Autodesk Fusion 360 part; units mm, degrees
sketch "podklad" plane through (0, 0, 0) normal (0, 1, 0) x (1, 0, 0)
  line L0 (45, -67.4927) -> (75, -67.4927) construction
  line L1 (-75.0372, -23.4927) -> (-85, -23.4927)
  arc A0 (96.7123, 33.4364) -> (98.5902, 36.1245) centre (96.7123, 35.4364) ccw
  line L2 (45, -38.4927) -> (45, -67.4927) construction
  line L3 (85, -33.4277) -> (85, -23.4927)
  line L4 (-75.0372, -23.4927) -> (-75.0372, 23.5073)
  line L5 (74.9628, -23.4927) -> (74.9628, 23.5073)
  line L6 (0, 105) -> (0, -105) construction
  line L7 (-85, 23.5073) -> (-75.0372, 23.5073)
  arc A1 (-98.5902, 36.1245) -> (-96.7123, 33.4364) centre (-96.7123, 35.4364) ccw
  arc A2 (-96.7154, -33.4277) -> (-98.5934, -36.1156) centre (-96.7154, -35.4277) ccw
  line L8 (74.9628, -23.4927) -> (85, -23.4927)
  line L9 (85, 23.5073) -> (74.9628, 23.5073)
  line L10 (-85, 33.4364) -> (-85, 23.5073)
  arc A3 (-98.5934, -36.1156) -> (98.5934, -36.1156) centre (0, 0) ccw
  line L11 (85, 33.4364) -> (85, 23.5073)
  line L12 (96.7123, 33.4364) -> (85, 33.4364)
  line L13 (-96.7154, -33.4277) -> (-85, -33.4277)
  arc A4 (98.5934, -36.1156) -> (96.7154, -33.4277) centre (96.7154, -35.4277) ccw
  line L14 (75, -67.4927) -> (75, -38.4927) construction
  arc A5 (98.5902, 36.1245) -> (15, 103.923) centre (0, 0) ccw
  arc A6 (15, 103.923) -> (-15, 103.923) centre (0, 0) ccw
  arc A7 (-15, 103.923) -> (-98.5902, 36.1245) centre (0, 0) ccw
  circle A8 centre (75, -38.4927) radius 1.1
  line L15 (75, -38.4927) -> (45, -38.4927) construction
  line L16 (-96.7123, 33.4364) -> (-85, 33.4364)
  circle A9 centre (75, -67.4927) radius 1.1
  circle A10 centre (45, -38.4927) radius 1.1
  line L17 (96.7154, -33.4277) -> (85, -33.4277)
  line L18 (-85, -33.4277) -> (-85, -23.4927)
  circle A11 centre (45, -67.4927) radius 1.1
  line L19 (51, -45) -> (69, -45)
  line L20 (70, -46) -> (70, -62)
  line L21 (69, -63) -> (51, -63)
  line L22 (50, -62) -> (50, -46)
  circle A12 centre (-30, -94.9953) radius 1.85
  circle A13 centre (30, -94.9953) radius 1.85
  circle A14 centre (-29.9934, 95.0047) radius 1.85
  circle A15 centre (29.9934, 95.0047) radius 1.85
  circle A16 centre (0, 0) radius 10
  circle A17 centre (-20, 0.003) radius 1.85
  circle A18 centre (-30, 0.0036) radius 1.85
  circle A19 centre (-40, 0.0023) radius 1.85
  circle A20 centre (-50, 0.0036) radius 1.85
  circle A21 centre (50, 0.0036) radius 1.85
  circle A22 centre (40, 0.0023) radius 1.85
  circle A23 centre (30, 0.0036) radius 1.85
  circle A24 centre (20, 0.003) radius 1.85
  arc A25 (51, -45) -> (50, -46) centre (51, -46) ccw
  arc A26 (70, -46) -> (69, -45) centre (69, -46) ccw
  arc A27 (69, -63) -> (70, -62) centre (69, -62) ccw
  arc A28 (50, -62) -> (51, -63) centre (51, -62) ccw
  line L23 (2.5, 0) -> (20, 0)
  line L24 (6, 15) -> (29, 15)
  line L25 (30, 16) -> (30, 74)
  line L26 (29, 75) -> (6, 75)
  line L27 (5, 74) -> (5, 16)
  arc A29 (6, 75) -> (5, 74) centre (6, 74) ccw
  arc A30 (30, 74) -> (29, 75) centre (29, 74) ccw
  arc A31 (29, 15) -> (30, 16) centre (29, 16) ccw
  arc A32 (5, 16) -> (6, 15) centre (6, 16) ccw
  line L28 (-56.6497, 57.6211) -> (-52.6497, 57.6211)
  line L29 (-52.6497, 33.6211) -> (-56.6497, 33.6211)
  line L30 (-56.6497, 33.6211) -> (-56.6497, 35.202)
  line L31 (-56.6497, 54.798) -> (-56.6497, 57.6211)
  line L32 (-52.6497, 57.6211) -> (-52.6497, 54.798)
  line L33 (-52.6497, 35.202) -> (-52.6497, 33.6211)
  arc A33 (-56.6497, 54.798) -> (-56.6497, 35.202) centre (-54.6497, 45) ccw
  arc A34 (-52.6497, 35.202) -> (-52.6497, 54.798) centre (-54.6497, 45) ccw
  point P0 (-7.5, -102.9967)
  point P1 (-82.0372, 22.8073)
  point P2 (-17.0372, -22.7927)
  point P3 (81.9628, 22.8073)
  point P4 (-0.0372, 0.0073)
  point P5 (-82.0372, -22.7927)
  point P6 (16.9628, 27.0073)
  point P7 (16.9628, 22.8073)
  point P8 (-17.0372, 27.0073)
  point P9 (16.9628, -22.7927)
  point P10 (81.9628, -22.7927)
  point P11 (16.9628, -26.9927)
  dimension "d1" = 210
  dimension "d2" = 2
  dimension "d3" = 2
  dimension "d4" = 2
  dimension "d5" = 2
  dimension "d26" = 30
  dimension "d27" = 29
  dimension "d28" = 2.2
  dimension "d29" = 2.2
  dimension "d30" = 2.2
  dimension "d31" = 2.2
  dimension "d32" = 45
  dimension "d33" = 15
  dimension "d39" = 3.7
  dimension "d40" = 20
  dimension "d41" = 3.7
  dimension "d42" = 3.7
  dimension "d43" = 3.7
  dimension "d44" = 20
  dimension "d45" = 30
  dimension "d46" = 40
  dimension "d47" = 3.7
  dimension "d48" = 50
  dimension "d49" = 1
  dimension "d50" = 1
  dimension "d51" = 1
  dimension "d52" = 1
  dimension "d74" = 1
  dimension "d75" = 20
  dimension "d76" = 4
  dimension "d77" = 24
  dimension "d78" = 2
extrude "Extrude1" add sketch "podklad" along normal blind 5
sketch "diry_hlavy_sroubu" plane through (0, 5, 0) normal (0, 1, 0) x (-1, 0, 0)
  circle A0 centre (29.9934, -95.0047) radius 1.85
  circle A1 centre (-29.9934, -95.0047) radius 1.85
  circle A2 centre (0, 0) radius 10
  circle A3 centre (40, -0.0023) radius 1.85
  circle A4 centre (-30, -0.0036) radius 1.85
  circle A5 centre (30, -0.0036) radius 1.85
  arc A6 (-51, 45) -> (-50, 46) centre (-51, 46) ccw
  line L0 (-51, 45) -> (-69, 45)
  arc A7 (-70, 46) -> (-69, 45) centre (-69, 46) ccw
  line L1 (-70, 46) -> (-70, 62)
  arc A8 (-69, 63) -> (-70, 62) centre (-69, 62) ccw
  line L2 (-69, 63) -> (-51, 63)
  arc A9 (-50, 62) -> (-51, 63) centre (-51, 62) ccw
  line L3 (-50, 62) -> (-50, 46)
  circle A10 centre (-45, 67.4927) radius 1.1
  circle A11 centre (-30, 94.9953) radius 1.85
  circle A12 centre (-50, -0.0036) radius 1.85
  circle A13 centre (-45, 38.4927) radius 1.1
  circle A14 centre (-75, 67.4927) radius 1.1
  circle A15 centre (50, -0.0036) radius 1.85
  circle A16 centre (30, 94.9953) radius 1.85
  circle A17 centre (-40, -0.0023) radius 1.85
  circle A18 centre (-20, -0.003) radius 1.85
  circle A19 centre (20, -0.003) radius 1.85
  circle A20 centre (-75, 38.4927) radius 1.1
  arc A21 (96.7154, 33.4277) -> (98.5934, 36.1156) centre (96.7154, 35.4277) ccw
  arc A22 (98.5934, 36.1156) -> (-98.5934, 36.1156) centre (0, 0) ccw
  arc A23 (-98.5934, 36.1156) -> (-96.7154, 33.4277) centre (-96.7154, 35.4277) ccw
  line L4 (-96.7154, 33.4277) -> (-85, 33.4277)
  line L5 (-85, 33.4277) -> (-85, 23.4927)
  line L6 (-85, 23.4927) -> (-74.9628, 23.4927)
  line L7 (-74.9628, 23.4927) -> (-74.9628, -23.5073)
  line L8 (-74.9628, -23.5073) -> (-85, -23.5073)
  line L9 (-85, -23.5073) -> (-85, -33.4364)
  line L10 (-85, -33.4364) -> (-96.7123, -33.4364)
  arc A24 (-96.7123, -33.4364) -> (-98.5902, -36.1245) centre (-96.7123, -35.4364) ccw
  arc A25 (-98.5902, -36.1245) -> (98.5902, -36.1245) centre (0, 0) ccw
  arc A26 (98.5902, -36.1245) -> (96.7123, -33.4364) centre (96.7123, -35.4364) ccw
  line L11 (96.7123, -33.4364) -> (85, -33.4364)
  line L12 (85, -33.4364) -> (85, -23.5073)
  line L13 (85, -23.5073) -> (75.0372, -23.5073)
  line L14 (75.0372, -23.5073) -> (75.0372, 23.4927)
  line L15 (75.0372, 23.4927) -> (85, 23.4927)
  line L16 (85, 23.4927) -> (85, 33.4277)
  line L17 (85, 33.4277) -> (96.7154, 33.4277)
  circle A27 centre (29.9934, -95.0047) radius 3.5
  circle A28 centre (-29.9934, -95.0047) radius 3.5
  circle A29 centre (30, 94.9953) radius 3.5
  circle A30 centre (-30, 94.9953) radius 3.5
  line L18 (-5, -16) -> (-5, -74)
  line L19 (-6, -75) -> (-29, -75)
  line L20 (-30, -74) -> (-30, -16)
  line L21 (-29, -15) -> (-6, -15)
  arc A31 (-5, -16) -> (-6, -15) centre (-6, -16) ccw
  arc A32 (-6, -75) -> (-5, -74) centre (-6, -74) ccw
  arc A33 (-30, -74) -> (-29, -75) centre (-29, -74) ccw
  arc A34 (-29, -15) -> (-30, -16) centre (-29, -16) ccw
  line L22 (52.6497, -35.202) -> (52.6497, -33.6211)
  line L23 (52.6497, -33.6211) -> (56.6497, -33.6211)
  line L24 (56.6497, -33.6211) -> (56.6497, -35.202)
  arc A35 (56.6497, -54.798) -> (56.6497, -35.202) centre (54.6497, -45) ccw
  line L25 (56.6497, -54.798) -> (56.6497, -57.6211)
  line L26 (56.6497, -57.6211) -> (52.6497, -57.6211)
  line L27 (52.6497, -57.6211) -> (52.6497, -54.798)
  arc A36 (52.6497, -35.202) -> (52.6497, -54.798) centre (54.6497, -45) ccw
  dimension "d55" = 7
  dimension "d56" = 7
  dimension "d57" = 7
  dimension "d58" = 7
extrude "Extrude3" cut sketch "diry_hlavy_sroubu" against normal blind 3 contours A27 | A28 | A29 | A30
sketch "sloupky_displej" plane through (0, 5, 0) normal (0, 1, 0) x (-1, 0, 0)
  circle A0 centre (-45, 38.4927) radius 4
  circle A1 centre (-75, 38.4927) radius 4
  circle A2 centre (-45, 67.4927) radius 4
  circle A3 centre (-75, 67.4927) radius 4
  circle A4 centre (-45, 67.4927) radius 1.1
  circle A5 centre (-75, 67.4927) radius 1.1
  circle A6 centre (-75, 38.4927) radius 1.1
  circle A7 centre (-45, 38.4927) radius 1.1
  point P0 (-45, 38.4927)
  point P1 (-75, 38.4927)
  point P2 (-45, 67.4927)
  point P3 (-75, 67.4927)
  point P4 (-43.9, 67.4927)
  point P5 (-73.9, 67.4927)
  point P6 (-73.9, 38.4927)
  point P7 (-43.9, 38.4927)
  dimension "d63" = 8
  dimension "d64" = 8
  dimension "d65" = 8
  dimension "d66" = 8
extrude "Extrude4" add sketch "sloupky_displej" along normal blind 5
Input: part model. Units: mm. Frame: model coordinates. A direction names the side the tool comes from. Give positions to 0.01 mm unless a question says otherwise; leave off trailing zeros. Write each loop counter-clockwise with the first axis right and the second up, starting at its lowest first coordinate (ties: lowest second). Pieces come first, ordered by that corner, then holes.
Q1. Pull-direction query (X, two-part tool) for faces 4 (the face through (91, 2, -33.436)), 5 (the face through (50, 2, 54)), 6 (the face through (85, 2, -29)); classes: pulls with the +X half, pulls with the -X half, needs draft (parallel to the pull), parting line crosses it, or undercut.
Q2. Section C-C, the plane y = 3.5. State how many separate pieces and enclosed holes the cut face has, plus the area to 3 significant figures.
Q3. Section A-A, the plane x = 0. Output: boundary loops of the cut face in (y, z), plus the area to 3 significant figures.
Q4. Material intervals for probe 1 along Z at (x, y) = (-30, 3.6); probe 2 along Z at (x, y) = (20.5, 1.75); probe 3 along X at (y, z) = (2.75, 68), sorted ascending.
Q5. First-contact query: P1, Ø2, axis at y = 1, z = -33.5, coming from the +X side; P2, Ø5, axis at y = 2, z = 75, coming from the +X side; P3, Ø4, axis at x = -81, y = 1.5, coming from the -Z side. Flat tips, straight axial feed; report the tip coordinate or a pass-through.
Q6. Section D-D, the plane z = 20. Output: boundary loops of the cut face in (x, y), plus the area to 3 significant figures.
Q7. Set-up query: faces 1 (the face through (78.17, 7.46, 40.93)), 2 (the face through (17, 2, -15)), 3 (the face through (-75.037, 2, 0)). Return all of +Z, -Z, +X, -X, +Y, -Y with unobstructed straight access to the full face (end or side cutting, diameter ignored); none if empty.
Q8. Section B-B, the plane z = -6. Output: boundary loops of the cut face in (x, y).
Filled in:
1. face 4: needs draft
1. face 5: undercut
1. face 6: pulls with the +X half
2. separate pieces: 1
2. enclosed holes: 20
2. area: 28,500 mm2
3. outline: (0, -105) - (5, -105) - (5, -10) - (0, -10) - close; (0, 10) - (5, 10) - (5, 105) - (0, 105) - close
3. area: 950 mm2
4. probe 1: z = -100.62 to -98.5, -91.5 to -1.85, 1.85 to 91.5, 98.5 to 100.62
4. probe 2: z = -102.98 to -75, -15 to -1.78, 1.78 to 102.98
4. probe 3: x = -80.01 to 44.02, 45.98 to 74.02, 75.98 to 80.01
5. P1: stops at x = 98.48
5. P2: stops at x = 75.95
5. P3: stops at z = -69.17
6. outline: (-75.04, 0) - (74.96, 0) - (74.96, 5) - (-75.04, 5) - close
6. area: 750 mm2
7. face 1: +Y
7. face 2: +Y, -Y
7. face 3: -X, +Y, -Y
8. outline: (-75.04, 0) - (-8, 0) - (-8, 5) - (-75.04, 5) - close; (8, 0) - (74.96, 0) - (74.96, 5) - (8, 5) - close
